Build history of the part. All positions in model axes, mm. Give positions to 0.01 mm unless a question says otherwise; leave off trailing zeros. Order: outer loops, then holes, each group sorted by start corner. A loop starts at its lowest first (then second) coordinate and runs counter-clockwise, first axis right, second up. Notation, with made-up numbers: (27, -3.5) - (50, -3.5) arc R28 cw to (50, 18.5) - close; hole circle Ø3 at (42.5, -35.5). An arc over 180 degrees is marked (long way). Write each question's results on one line, items separated by ' | '. Start each with the question number.
from build123d import *

# Parameters (mm, degrees)
SKETCH1_W                 = 68.199
SKETCH1_H                 = 14.859
BOSS_EXTRUDE1_DEPTH       = 9.398
SKETCH2_W                 = 6.35
SKETCH2_H                 = 13.335
CUT_EXTRUDE1_DEPTH        = 70.649166736
F_5_CLEARANCE_HOLE1_D     = 3.556
F_5_CLEARANCE_HOLE1_DEPTH = 1.524
F_5_CLEARANCE_HOLE2_D     = 3.556
F_5_CLEARANCE_HOLE2_DEPTH = 14.859
F_5_CLEARANCE_HOLE3_D     = 3.556
FILLET1_R                 = 0.635


with BuildPart() as part:
    # Sketch1 → Boss-Extrude1 (new body)
    with BuildSketch(Plane(origin=(-4.699, 0, 0), x_dir=(0, -1, 0), z_dir=(-1, 0, 0))):
        with Locations((-34.0995, -5.9055)):
            Rectangle(SKETCH1_W, SKETCH1_H)
    extrude(amount=-BOSS_EXTRUDE1_DEPTH)

    # Sketch2 → Cut-Extrude1 (cut, through all)
    with BuildSketch(Plane.XZ):
        with Locations((0, -6.6675)):
            Rectangle(SKETCH2_W, SKETCH2_H)
    extrude(amount=-CUT_EXTRUDE1_DEPTH, mode=Mode.SUBTRACT)

    # #5 Clearance Hole1
    with Locations(Plane(origin=(4.699, 0, 0), x_dir=(0, 0, -1), z_dir=(1, 0, 0))):
        with Locations((8.5725, 53.6575), (8.5725, 63.4365), (8.5725, 43.8785), (8.5725, 34.0995), (8.5725, 24.3205), (8.5725, 14.5415), (8.5725, 4.7625)):
            Hole(F_5_CLEARANCE_HOLE1_D / 2, depth=F_5_CLEARANCE_HOLE1_DEPTH)

    # #5 Clearance Hole2
    with Locations(Plane.XY.offset(1.524)):
        with Locations((0, 53.6575), (0, 63.4365), (0, 43.8785), (0, 34.0995), (0, 24.3205), (0, 14.5415), (0, 4.7625)):
            Hole(F_5_CLEARANCE_HOLE2_D / 2, depth=F_5_CLEARANCE_HOLE2_DEPTH)

    # #5 Clearance Hole3 (through all)
    with Locations(Plane(origin=(-3.175, 0, 0), x_dir=(0, 0, -1), z_dir=(1, 0, 0))):
        with Locations((8.5725, 53.6575), (8.5725, 63.4365), (8.5725, 43.8785), (8.5725, 34.0995), (8.5725, 24.3205), (8.5725, 14.5415), (8.5725, 4.7625)):
            Hole(F_5_CLEARANCE_HOLE3_D / 2)

    # Fillet1
    fillet1_edges = [part.edges().sort_by_distance(p)[0] for p in [
        (-3.937, 68.199, -13.335),
        (-3.937, 0, -13.335),
        (3.937, 0, -13.335),
        (3.937, 68.199, -13.335),
    ]]
    fillet(fillet1_edges, radius=FILLET1_R)


solid = part.part
Item 1: Cut at A-A, the plane z = -12. List the corners of the cut face in (x, y) (3 decimals), then the cut area to 3 significant figures.
Item 2: Cut at C-C, the plane y = 28. List the corners of the cut face in (x, z) (3 decimals).
Item 3: Cut at B-B, the plane x = 0. Count the separate pieces of the cut face and the enclosed holes in it, then the cut area to 3 significant figures.
Item 4: Cut at D-D, the plane z = 0.75. List the corners of the cut face in (x, y), then the cut area to 3 significant figures.
Item 5: Flat gauge pin, fed straight in: pin 1 Ø4 at (x, y) = (0, 24.32) entering from -Z. Where does the tip first touch, or does it go through?
Item 6: Probe line 1 along X through (y, z) = (17.5, -11.5) (3 decimals); line 2 along Z through (x, y) = (-1.25, 16.5); line 3 along Z through (x, y) = (3.5, 4.5) (3 decimals). List the from-to ranges inside material, lowest first. Write a range as from..to.
Item 7: Two-plate mould, pull along Z, no slides. Class faces 1 (the flat face through (-4, 68.199, -4)), 2 (the flat face through (2, 34, 0)), 3 (the cylindrical face through (3.9, 65.2, -8.8)): +Z half, -Z half, draft (parallel to the pull), parting line (faces both ways), or undercut.
Values found:
1) outline: (-4.699, 0) - (-3.175, 0) - (-3.175, 68.199) - (-4.699, 68.199) - close; (3.175, 0) - (4.699, 0) - (4.699, 68.199) - (3.175, 68.199) - close | area: 208 mm2
2) outline: (-4.699, -13.335) - (-3.175, -13.335) - (-3.175, 0) - (3.175, 0) - (3.175, -13.335) - (4.699, -13.335) - (4.699, 1.524) - (-4.699, 1.524) - close
3) separate pieces: 8 | enclosed holes: 0 | area: 66.0 mm2
4) outline: (-4.7, 0) - (4.7, 0) - (4.7, 68.2) - (-4.7, 68.2) - close; hole circle Ø3.56 at (0, 4.76); hole circle Ø3.56 at (0, 14.54); hole circle Ø3.56 at (0, 24.32); hole circle Ø3.56 at (0, 34.1); hole circle Ø3.56 at (0, 43.88); hole circle Ø3.56 at (0, 53.66); hole circle Ø3.56 at (0, 63.44) | area: 571 mm2
5) pin 1: stops at z = 0
6) line 1: x = -4.699..-3.175, 3.175..4.699 | line 2: z = 0..1.52 | line 3: z = -13.335..-10.331, -6.814..1.524
7) face 1: draft | face 2: -Z half | face 3: undercut
